```python
from build123d import *

# Parameters (mm, degrees)
SKETCH1_W             = 80
SKETCH1_H             = 10
BOSS_EXTRUDE1_DEPTH   = 2
FILLET1_R             = 3
F_3_0MM_DOWEL_HOLE1_D = 3


with BuildPart() as part:
    # Sketch1 → Boss-Extrude1 (new body)
    with BuildSketch(Plane(origin=(0, 0, 0), x_dir=(1, 0, 0), z_dir=(0, 1, 0))):
        Rectangle(SKETCH1_W, SKETCH1_H)
    extrude(amount=BOSS_EXTRUDE1_DEPTH)

    # Fillet1
    fillet1_edges = [part.edges().sort_by_distance(p)[0] for p in [
        (40, 1, 5),
        (-40, 1, 5),
        (-40, 1, -5),
        (40, 1, -5),
    ]]
    fillet(fillet1_edges, radius=FILLET1_R)

    # Ø3.0mm Dowel Hole1 (through all)
    with Locations(Plane(origin=(0, 0, 0), x_dir=(-1, 0, 0), z_dir=(0, -1, 0))):
        with Locations((-34, 0), (21, 0)):
            Hole(F_3_0MM_DOWEL_HOLE1_D / 2)


solid = part.part
```
Could you check a few things on this model? Use its own coordinates, in mm. Round coordinates to 2 decimals unless told otherwise and drop trailing zeros. Write each loop counter-clockwise with the first axis right and the second up, starting at its lowest first coordinate (ties: lowest second). Pieces come first, ordered by that corner, then holes.
(1) Suppose I cut it at A-A on z = 0. Write out the boundary of the cut face in (x, y).
Findings below:
outline: (-40, 0) - (-22.5, 0) - (-22.5, 2) - (-40, 2) - close; (-19.5, 0) - (32.5, 0) - (32.5, 2) - (-19.5, 2) - close; (35.5, 0) - (40, 0) - (40, 2) - (35.5, 2) - close
(2) Suppose I cut it at C-C on x = 34. Write out the boundary of the cut face in (y, z), and give its area (3 significant figures).
Findings below:
outline: (0, -5) - (2, -5) - (2, -1.5) - (0, -1.5) - close; (0, 1.5) - (2, 1.5) - (2, 5) - (0, 5) - close
area: 14.0 mm2
(3) If I drill on probe 1 along X at (y, z) = (1.7, -1); probe 2 along X at (y, z) = (1.9, -0.25); probe 3 along Z at (x, y) = (34, 1.35), over which ranges is the centre line in solid material (lowest first)?
Findings below:
probe 1: x = -40 to -22.12, -19.88 to 32.88, 35.12 to 40
probe 2: x = -40 to -22.48, -19.52 to 32.52, 35.48 to 40
probe 3: z = -5 to -1.5, 1.5 to 5
(4) Thinking about a two-plate mould opening in Z: for faces 1 (the face through (-1, 1, 5)), 2 (the face through (-22.5, 1.01, -0.07)), 3 (the face through (-40, 1, 0)), which applies, +Z half, -Z half, draft (parallel to the pull), parting line (faces both ways), or undercut?
Findings below:
face 1: +Z half
face 2: undercut
face 3: draft
(5) For pin 1 (2.5 mm diameter, centred on x = -21, z = 0, fed in from +Y); pin 2 (6 mm diameter, centred on x = -16.5, z = -1.5, fed in from -Y), each with a flat end and sliding along its axis, tell me the tip position at first contact or that it passes through.
Findings below:
pin 1: passes through
pin 2: stops at y = 0
(6) Suppose I cut it at B-B on y = 1.55. Write out the boundary of the cut face in (x, z).
Findings below:
outline: (-40, -2) arc R3 ccw to (-37, -5) - (37, -5) arc R3 ccw to (40, -2) - (40, 2) arc R3 ccw to (37, 5) - (-37, 5) arc R3 ccw to (-40, 2) - close; hole circle Ø3 at (-21, 0); hole circle Ø3 at (34, 0)
